Can you work these out from the model? Positions are in its coordinate system, mm. A direction names the side the tool comes from. Give positions to 0.01 mm unless a question says otherwise; leave off trailing zeros. Order: outer loops, then holes, each group sorted by start corner. A loop starts at its lowest first (then second) coordinate and runs counter-clockwise, first axis right, second up. Notation, with made-up numbers: (39, 71.5) - (60, 71.5) arc R18 cw to (60, 80.5) - close; hole circle Ø4 at (3, -28). An arc over 180 degrees is marked (long way). One line per question, with ' | ' between items.
```python
from build123d import *

# Parameters (mm, degrees)
EXTRUDE_1_DEPTH     = 6
CUT_EXTRUDE_1_DEPTH = 4.5


with BuildPart() as part:
    # 草图1 → 凸台-拉伸1 (new body)
    with BuildSketch(Plane(origin=(0, 0, 0), x_dir=(1, 0, 0), z_dir=(0, 1, 0))):
        Polygon((-35, 0), (0, 0), (0, -40), (-6, -33.142857143), (-6, -16), (-16, -6), (-29.75, -6), align=None)
    extrude(amount=EXTRUDE_1_DEPTH)

    # 草图3 → 切除-拉伸1 (cut)
    with BuildSketch(Plane(origin=(0, 6, 0), x_dir=(1, 0, 0), z_dir=(0, 1, 0))):
        Polygon((-30.592463547, -2), (-28.842463547, -4), (-15.171572875, -4), (-4, -15.171572875), (-4, -32.391386911), (-2, -34.677101196), (-2, -2), align=None)
    extrude(amount=-CUT_EXTRUDE_1_DEPTH, mode=Mode.SUBTRACT)


solid = part.part
```
(1) Imagine slicing it at A-A (y = 5.3). List the corners of the cut face in (x, z) for me.
Answer below:
outline: (-35, 0) - (0, 0) - (0, 40) - (-6, 33.14) - (-6, 16) - (-16, 6) - (-29.75, 6) - close; hole (-30.59, 2) - (-2, 2) - (-2, 34.68) - (-4, 32.39) - (-4, 15.17) - (-15.17, 4) - (-28.84, 4) - close
(2) Imagine slicing it at C-C (z = 28). List the corners of the cut face in (x, y) for me, and give its area (3 significant figures).
Answer below:
outline: (-6, 0) - (0, 0) - (0, 6) - (-2, 6) - (-2, 1.5) - (-4, 1.5) - (-4, 6) - (-6, 6) - close | area: 27.0 mm^2
(3) If we mould it in two halves opening along X, with no side actions, what happens to faces 4 (the face through (-6, 3, 25)), 5 (the face through (0, 3, 20)), 6 (the face through (-7, 6, 14)), 7 (the face through (-16, 4, 2))? For each: released by +X, released by -X, zero draft, split by the parting line, or undercut.
Answer below:
face 4: released by -X | face 5: released by +X | face 6: zero draft | face 7: undercut
(4) Imagine slicing it at B-B (x = -19). List the corners of the cut face in (y, z) for me.
Answer below:
outline: (0, 0) - (6, 0) - (6, 2) - (1.5, 2) - (1.5, 4) - (6, 4) - (6, 6) - (0, 6) - close
(5) On a 3-axis mill with a long thin cutter (end or side, diameter ignored), from which of +Z, -Z, +X, -X, +Y, -Y can I reach the whole of each face in a straight line? I mean faces 1 (the face through (-10, 0, 10)), 2 (the face through (-23, 3, 6)), 3 (the face through (-22, 4, 4)). Say none if no direction works.
Answer below:
face 1: +Z, -Z, +X, -X, -Y | face 2: +Z, -X, +Y, -Y | face 3: +Y
(6) If I drill on line 1 (X direction, y = 3.8, z = 24.5); line 2 (Z direction, x = -22, y = 4.75); line 3 (Y direction, x = -28.5, z = 2.5), over which ranges is the centre line in solid material (lowest first)?
Answer below:
line 1: -6 to -4, -2 to 0 | line 2: 0 to 2, 4 to 6 | line 3: 0 to 1.5
(7) Will these pins go through, and if not, where does the flat tip stop? pin 1 (1.5 mm diameter, centred on x = -25.5, y = 2.5, fed in from +Z); pin 2 (3.5 mm diameter, centred on y = 3, z = 25.5, fed in from -X).
Answer below:
pin 1: z = 6 | pin 2: x = -6
